Design review of the part built by this model. Coordinates are the model's own, in mm. Coordinates: 2 decimals unless noted, no trailing zeros. Loops run counter-clockwise (first coordinate to the right, second up) from the corner with the lowest first, then second, coordinate; pieces in that order, holes last. Notation, with made-up numbers: M -9.75,-5 L 20.25,-5 A23 ccw 20.25,34 Z; hole C 51.25,60 d2. An arc over 180 degrees is marked long. Put each result on its own line as item: value. Start each with the question number.
(1) The part is to be moulded in two halves that separate along Y. For faces 1 (the flat face through (0, 0, 0.9)), 2 (the flat face through (0, 32.75, 0)), 3 (the cylindrical face through (-0.651, 14.957, 0.013)), say which applies: +Y half, -Y half, draft (parallel to the pull), parting line (faces both ways), or undercut.
(2) Clearance check with a flat-ended pin moving along its axis: pin 1 (8 mm diameter, centred on x = 0, y = 10, fed in from +Z). State where the tip first meets the part, or that it passes through.
(3) Take a section at C-C, the plane z = 0.1. Give the boundary of the cut face in (x, y).
(4) For probe 1 along Y at (x, z) = (0, 0.45); probe 2 along X at (y, z) = (12, 0.2); probe 3 along Y at (x, z) = (-1.5, 0.45), list the stretches that pass through material, from the lowest coordinate up. Write a range as [from, to].
(5) Take a section at B-B, the plane y = 10. Give the boundary of the cut face in (x, z).
(6) Take a section at A-A, the plane x = 0. Give the boundary of the cut face in (y, z), then the cut area to 3 significant figures.
```python
from build123d import *

# Parameters (mm, degrees)
SKETCH1_W           = 62
SKETCH1_H           = 65.5
BOSS_EXTRUDE1_DEPTH = 0.9
SKETCH2_R           = 5
CUT_EXTRUDE1_DEPTH  = 46.130948361


with BuildPart() as part:
    # Sketch1 → Boss-Extrude1 (new, symmetric)
    with BuildSketch(Plane.XY):
        Rectangle(SKETCH1_W, SKETCH1_H)
    extrude(amount=BOSS_EXTRUDE1_DEPTH, both=True)

    # Sketch2 → Cut-Extrude1 (cut, through all)
    with BuildSketch(Plane.XY.offset(0.9)):
        with Locations((0, 10)):
            Circle(SKETCH2_R)
    extrude(amount=-CUT_EXTRUDE1_DEPTH, mode=Mode.SUBTRACT)


solid = part.part
```
Computed values:
1. face 1: draft
1. face 2: +Y half
1. face 3: undercut
2. pin 1: passes through
3. outline: M -31,-32.75 L 31,-32.75 L 31,32.75 L -31,32.75 Z; hole C 0,10 d10
4. probe 1: y = [-32.75, 5], [15, 32.75]
4. probe 2: x = [-31, -4.58], [4.58, 31]
4. probe 3: y = [-32.75, 5.23], [14.77, 32.75]
5. outline: M -31,-0.9 L -5,-0.9 L -5,0.9 L -31,0.9 Z; M 5,-0.9 L 31,-0.9 L 31,0.9 L 5,0.9 Z
6. outline: M -32.75,-0.9 L 5,-0.9 L 5,0.9 L -32.75,0.9 Z; M 15,-0.9 L 32.75,-0.9 L 32.75,0.9 L 15,0.9 Z
6. area: 99.9 mm^2
